```python
from build123d import *

# Parameters (mm, degrees)
SKETCH_1_W          = 150
SKETCH_1_H          = 150
EXTRUDE_1_DEPTH     = 100
SKETCH_4_R          = 25
EXTRUDE_2_DEPTH     = 0.4
SKETCH_5_W          = 145
SKETCH_5_H          = 140
CUT_EXTRUDE_1_DEPTH = 95
SKETCH_7_W          = 10
SKETCH_7_H          = 10
EXTRUDE_3_DEPTH     = 5
EXTRUDE_4_DEPTH     = 5
SKETCH_10_W         = 10
SKETCH_10_H         = 10
EXTRUDE_5_DEPTH     = 5
EXTRUDE_6_DEPTH     = 5


with BuildPart() as part:
    # 草图1 → 凸台-拉伸1 (new body)
    with BuildSketch(Plane(origin=(0, 0, 0), x_dir=(1, 0, 0), z_dir=(0, 1, 0))):
        with Locations((-43.129330254, -16.974595843)):
            Rectangle(SKETCH_1_W, SKETCH_1_H)
    extrude(amount=EXTRUDE_1_DEPTH)

    # 草图4 → 凸台-拉伸2 (add)
    with BuildSketch(Plane(origin=(0, 100, 0), x_dir=(1, 0, 0), z_dir=(0, 1, 0))):
        with Locations(Location((-68.129330254, -16.974595843, 0), (0, 0, 270))):
            Circle(SKETCH_4_R)
    extrude(amount=EXTRUDE_2_DEPTH)

    # 草图5 → 切除-拉伸1 (cut)
    with BuildSketch(Plane.XZ):
        with Locations((-40.629330254, 16.974595843)):
            Rectangle(SKETCH_5_W, SKETCH_5_H)
    extrude(amount=-CUT_EXTRUDE_1_DEPTH, mode=Mode.SUBTRACT)

    # 草图7 → 凸台-拉伸3 (add)
    with BuildSketch(Plane.XY.offset(91.974595843)):
        with Locations((36.870669746, 50)):
            Rectangle(SKETCH_7_W, SKETCH_7_H)
    extrude(amount=-EXTRUDE_3_DEPTH)

    # 草图9 → 凸台-拉伸4 (add)
    with BuildSketch(Plane.XY.offset(91.974595843)):
        Polygon((31.870669746, 55), (41.870669746, 65), (41.870669746, 55), align=None)
        Polygon((31.870669746, 45), (41.870669746, 45), (41.870669746, 35), align=None)
    extrude(amount=-EXTRUDE_4_DEPTH)

    # 草图10 → 凸台-拉伸5 (add)
    with BuildSketch(Plane(origin=(0, 0, -58.025404157), x_dir=(-1, 0, 0), z_dir=(0, 0, -1))):
        with Locations((-36.870669746, 50)):
            Rectangle(SKETCH_10_W, SKETCH_10_H)
    extrude(amount=-EXTRUDE_5_DEPTH)

    # 草图11 → 凸台-拉伸6 (add)
    with BuildSketch(Plane(origin=(0, 0, -58.025404157), x_dir=(-1, 0, 0), z_dir=(0, 0, -1))):
        Polygon((-31.870669746, 55), (-41.870669746, 65), (-41.870669746, 55), align=None)
        Polygon((-31.870669746, 45), (-41.870669746, 45), (-41.870669746, 35), align=None)
    extrude(amount=-EXTRUDE_6_DEPTH)


solid = part.part
```
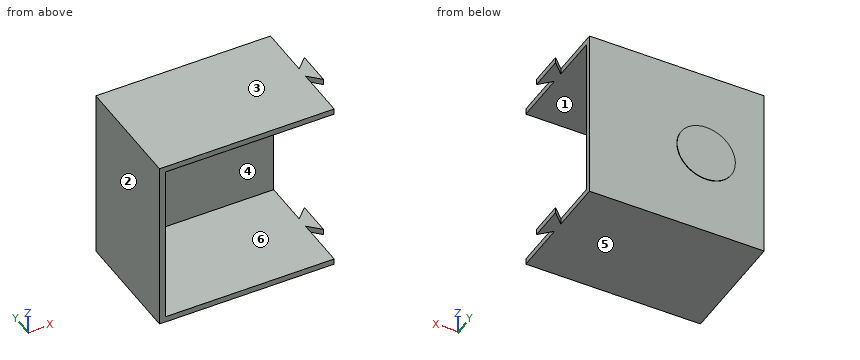
Can you work these out from the model? Positions are in its coordinate system, mm. Face numbers are marked on the shaded views. A direction names the side the tool comes from. Round coordinates to 2 decimals unless told otherwise and drop trailing zeros. Loops run counter-clockwise (first coordinate to the right, second up) from the corner with the lowest first, then second, coordinate; pieces in that order, holes last. Notation, with made-up numbers: M 74.25,11.25 L 85.25,11.25 A28 cw 85.25,50.25 Z; hole C 42.25,65.25 d7. An arc over 180 degrees is marked long. Answer in a Markdown table with one row per item.
1. If we section it at A-A, the plane x = -96: Please give me the cut outline in (y, z).
Established:
| item | result |
|---|---|
| outline | M 0,-58.03 L 100,-58.03 L 100,91.97 L 0,91.97 L 0,86.97 L 95,86.97 L 95,-53.03 L 0,-53.03 Z |
2. Please list where these lines run through material, in increasing order: line 1 (Z direction, x = -94.5, y = 25.5); line 2 (X direction, y = 26, z = 73); line 3 (Y direction, x = -85.5, z = 32). Write a range as from..to.
Established:
| item | result |
|---|---|
| line 1 | -58.03..-53.03, 86.97..91.97 |
| line 2 | -118.13..-113.13 |
| line 3 | 95..100.4 |
3. If we section it at B-B, the plane y = 41: Please give me the cut outline in (x, z).
Established:
| item | result |
|---|---|
| outline | M -118.13,-58.03 L 31.87,-58.03 L 31.87,-53.03 L -113.13,-53.03 L -113.13,86.97 L 31.87,86.97 L 31.87,91.97 L -118.13,91.97 Z; M 35.87,-58.03 L 41.87,-58.03 L 41.87,-53.03 L 35.87,-53.03 Z; M 35.87,86.97 L 41.87,86.97 L 41.87,91.97 L 35.87,91.97 Z |
4. If we section it at D-D, the plane y = 8: Please give me the cut outline in (x, z), plus the area to 3 significant figures.
Established:
| item | result |
|---|---|
| outline | M -118.13,-58.03 L 31.87,-58.03 L 31.87,-53.03 L -113.13,-53.03 L -113.13,86.97 L 31.87,86.97 L 31.87,91.97 L -118.13,91.97 Z |
| area | 2,200 mm² |
5. If we section it at C-C, the plane z = -25.5: Please give me the cut outline in (x, y).
Established:
| item | result |
|---|---|
| outline | M -118.13,0 L -113.13,0 L -113.13,95 L 31.87,95 L 31.87,100 L -118.13,100 Z |
6. On a 3-axis mill with a long thin cutter (end or side, diameter ignored), from which of +Z, -Z, +X, -X, +Y, -Y can I reach the whole of each face in a straight line? I mean the marked faces 5 and 6. Say none if no direction works.
Established:
| item | result |
|---|---|
| face 5 | -Z, +X, -X, +Y, -Y |
| face 6 | +X, -Y |
7. Thinking about a two-plate mould opening in Z: for the marked faces 1, 2, 3 and 4, which applies, pulls with the +Z half, pulls with the -Z half, needs draft (parallel to the pull), parting line crosses it, or undercut?
Established:
| item | result |
|---|---|
| face 1 | undercut |
| face 2 | needs draft |
| face 3 | pulls with the +Z half |
| face 4 | undercut |
8. I'm going to push flat-ended pins straight in: pin 1 Ø5 at (x, z) = (-33, 35) entering from +Y; pin 2 Ø10 at (y, z) = (84.5, 21.5) entering from +X; pin 3 Ø2.5 at (y, z) = (11.5, -55.5) entering from +X. Where does each tip first touch, or does it pass through?
Established:
| item | result |
|---|---|
| pin 1 | y = 100 |
| pin 2 | x = -113.13 |
| pin 3 | x = 31.87 |
